Source: CAD feature listing. Evaluate the final solid. Frame: model axes, mm. A direction names the side the tool comes from. Give positions to 0.01 mm unless a question says otherwise; leave off trailing zeros. Order: outer loops, then holes, each group sorted by start corner. A loop starts at its lowest first (then second) coordinate and runs counter-clockwise, first axis right, second up. Notation, with made-up numbers: M 20,48 L 53,48 A27 ccw 53,76 Z; hole C 69.5,-14.75 d9. An arc over 180 degrees is marked long. Return JSON: item names as keys, results as strings.
from build123d import *

# Parameters (mm, degrees)
F1_DEPTH     = 25.4
F2_T         = -2.54
F3_T4_DEPTH  = 109.6353324848
F3_T9_DEPTH  = 109.6353324848
F3_T14_DEPTH = 38.5537016023
F3_T19_DEPTH = 38.5537016023
F3_T24_DEPTH = 109.6353324848
F3_T29_DEPTH = 38.5537016023
F3_T34_DEPTH = 109.6353324848
F3_T39_DEPTH = 38.5537016023
F4_W         = 7.5721852481
F4_H         = 7.5721852481
F5_DEPTH     = 50.8
F6_SIZE      = 5.08
F7_R         = 5.08


# Not quite as in the source:
# - a fillet or chamfer that OpenCascade refuses, or shapes differently, is made with other operations: its cross-section is extruded or revolved along the edge and cut away or added


with BuildPart() as f1:
    # F0 (on Front) → F1 (new body)
    with BuildSketch(Plane.XZ):
        Polygon((-50.8, -50.8), (50.8, -50.8), (50.8, 50.8), (32.1275666356, 46.4897789061), (20.0797300786, -40.3164364398), (-20.0797300786, -40.3164364398), (-32.1275666356, 46.4897789061), (-50.8, 50.8), align=None)
    extrude(amount=F1_DEPTH)

    # F2
    f2_openings = [f1.faces().sort_by_distance(p)[0] for p in [
        (-41.463783, -12.7, 48.644889),
        (-26.103648, -12.7, 3.086671),
        (0, -12.7, -40.316436),
        (41.463783, -12.7, 48.644889),
        (26.103648, -12.7, 3.086671),
    ]]
    offset(amount=F2_T, openings=f2_openings)

    # F3: fillet of radius 5.08 on 8 edges, made by hand


with BuildPart() as f3_tool2:
    # F3_s3 → F3_t4 (new body)
    with BuildSketch(Plane(origin=(8.4495366949, 0, 60.8800010222), x_dir=(0, 1, 0), z_dir=(-0.1374722959, 0, -0.9905056122))):
        with BuildLine():
            ThreePointArc((0, 25.4314784161), (-1.8594090512, 27.2908874673), (-2.54, 29.8308874673))
            Line((-2.54, 29.8308874673), (-2.54, 25.4314784161))
            Line((-2.54, 25.4314784161), (0, 25.4314784161))
        make_face()
    extrude(amount=F3_T4_DEPTH)

    split(bisect_by=Plane.XY.offset(-40.3164364398), keep=Keep.TOP)


with BuildPart() as f1_1:
    add(f1.part)

    # F3_t1: cut F3_tool2
    add(f3_tool2.part, mode=Mode.SUBTRACT)


with BuildPart() as f3_tool7:
    # F3_s8 → F3_t9 (new body)
    with BuildSketch(Plane(origin=(6.6222841773, 0, -47.7144111022), x_dir=(0, 1, 0), z_dir=(-0.1374722959, 0, 0.9905056122))):
        with BuildLine():
            ThreePointArc((0, 25.4314784161), (-1.8594090512, 27.2908874673), (-2.54, 29.8308874673))
            Line((-2.54, 29.8308874673), (-2.54, 25.4314784161))
            Line((-2.54, 25.4314784161), (0, 25.4314784161))
        make_face()
    extrude(amount=F3_T9_DEPTH)

    split(bisect_by=Plane.XY.offset(-40.3164364398), keep=Keep.TOP)


with BuildPart() as f1_2:
    add(f1_1.part)

    # F3_t6: cut F3_tool7
    add(f3_tool7.part, mode=Mode.SUBTRACT)


with BuildPart() as f3_tool12:
    # F3_s13 → F3_t14 (new body)
    with BuildSketch(Plane(origin=(67.5399359806, 0, 15.5904723858), x_dir=(0, 1, 0), z_dir=(-0.9743774967, 0, -0.2249188607))):
        with BuildLine():
            ThreePointArc((0, -38.0724987065), (-1.8594090512, -36.2130896553), (-2.54, -33.6730896553))
            Line((-2.54, -33.6730896553), (-2.54, -38.0724987065))
            Line((-2.54, -38.0724987065), (0, -38.0724987065))
        make_face()
    extrude(amount=F3_T14_DEPTH)

    split(bisect_by=Plane.YZ.offset(48.26), keep=Keep.BOTTOM)


with BuildPart() as f1_3:
    add(f1_2.part)

    # F3_t11: cut F3_tool12
    add(f3_tool12.part, mode=Mode.SUBTRACT)


with BuildPart() as f3_tool17:
    # F3_s18 → F3_t19 (new body)
    with BuildSketch(Plane(origin=(-29.9740767247, 0, 6.9190177438), x_dir=(0, 1, 0), z_dir=(-0.9743774967, 0, 0.2249188607))):
        with BuildLine():
            ThreePointArc((0, -38.0724987065), (-1.8594090512, -36.2130896553), (-2.54, -33.6730896553))
            Line((-2.54, -33.6730896553), (-2.54, -38.0724987065))
            Line((-2.54, -38.0724987065), (0, -38.0724987065))
        make_face()
    extrude(amount=F3_T19_DEPTH)

    split(bisect_by=Plane.YZ.offset(-48.26), keep=Keep.TOP)


with BuildPart() as f1_4:
    add(f1_3.part)

    # F3_t16: cut F3_tool17
    add(f3_tool17.part, mode=Mode.SUBTRACT)


with BuildPart() as f3_tool22:
    # F3_s23 → F3_t24 (new body)
    with BuildSketch(Plane(origin=(6.6222841773, 0, -47.7144111022), x_dir=(0, 1, 0), z_dir=(-0.1374722959, 0, 0.9905056122))):
        with BuildLine():
            ThreePointArc((-25.4, 25.4314784161), (-23.5405909488, 27.2908874673), (-22.86, 29.8308874673))
            Line((-22.86, 29.8308874673), (-22.86, 25.4314784161))
            Line((-22.86, 25.4314784161), (-25.4, 25.4314784161))
        make_face()
    extrude(amount=F3_T24_DEPTH)

    split(bisect_by=Plane.XY.offset(-40.3164364398), keep=Keep.TOP)


with BuildPart() as f1_5:
    add(f1_4.part)

    # F3_t21: cut F3_tool22
    add(f3_tool22.part, mode=Mode.SUBTRACT)


with BuildPart() as f3_tool27:
    # F3_s28 → F3_t29 (new body)
    with BuildSketch(Plane(origin=(-29.9740767247, 0, 6.9190177438), x_dir=(0, 1, 0), z_dir=(-0.9743774967, 0, 0.2249188607))):
        with BuildLine():
            ThreePointArc((-25.4, -38.0724987065), (-23.5405909488, -36.2130896553), (-22.86, -33.6730896553))
            Line((-22.86, -33.6730896553), (-22.86, -38.0724987065))
            Line((-22.86, -38.0724987065), (-25.4, -38.0724987065))
        make_face()
    extrude(amount=F3_T29_DEPTH)

    split(bisect_by=Plane.YZ.offset(-48.26), keep=Keep.TOP)


with BuildPart() as f1_6:
    add(f1_5.part)

    # F3_t26: cut F3_tool27
    add(f3_tool27.part, mode=Mode.SUBTRACT)


with BuildPart() as f3_tool32:
    # F3_s33 → F3_t34 (new body)
    with BuildSketch(Plane(origin=(8.4495366949, 0, 60.8800010222), x_dir=(0, 1, 0), z_dir=(-0.1374722959, 0, -0.9905056122))):
        with BuildLine():
            ThreePointArc((-25.4, 25.4314784161), (-23.5405909488, 27.2908874673), (-22.86, 29.8308874673))
            Line((-22.86, 29.8308874673), (-22.86, 25.4314784161))
            Line((-22.86, 25.4314784161), (-25.4, 25.4314784161))
        make_face()
    extrude(amount=F3_T34_DEPTH)

    split(bisect_by=Plane.XY.offset(-40.3164364398), keep=Keep.TOP)


with BuildPart() as f1_7:
    add(f1_6.part)

    # F3_t31: cut F3_tool32
    add(f3_tool32.part, mode=Mode.SUBTRACT)


with BuildPart() as f3_tool37:
    # F3_s38 → F3_t39 (new body)
    with BuildSketch(Plane(origin=(67.5399359806, 0, 15.5904723858), x_dir=(0, 1, 0), z_dir=(-0.9743774967, 0, -0.2249188607))):
        with BuildLine():
            ThreePointArc((-25.4, -38.0724987065), (-23.5405909488, -36.2130896553), (-22.86, -33.6730896553))
            Line((-22.86, -33.6730896553), (-22.86, -38.0724987065))
            Line((-22.86, -38.0724987065), (-25.4, -38.0724987065))
        make_face()
    extrude(amount=F3_T39_DEPTH)

    split(bisect_by=Plane.YZ.offset(48.26), keep=Keep.BOTTOM)


with BuildPart() as f1_8:
    add(f1_7.part)

    # F3_t36: cut F3_tool37
    add(f3_tool37.part, mode=Mode.SUBTRACT)

    # F4 (on Front) → F5 (join)
    with BuildSketch(Plane.XZ):
        Polygon((-73.3337104321, -50.8196800947), (-54.8367798328, -50.8196800947), (-54.8367798328, -43.2474948466), (-47.2645945847, -43.2474948466), (-47.2645945847, -30.0912298262), (-73.3337104321, -30.0912298262), align=None)
        with Locations((-51.0506872088, -47.0335874707)):
            Rectangle(F4_W, F4_H)
    extrude(amount=F5_DEPTH)

    # F6
    f6_edges = [f1_8.edges().sort_by_distance(p)[0] for p in [
        (-50.8, -12.7, -30.09123),
    ]]
    chamfer(f6_edges, length=F6_SIZE)

    # F7
    f7_edges = [f1_8.edges().sort_by_distance(p)[0] for p in [
        (-73.33371, -25.4, -30.09123),
        (-60.299153, -50.8, -50.81968),
    ]]
    fillet(f7_edges, radius=F7_R)


solid = f1_8.part
1. First-contact query: pin 1 (5 mm diameter, centred on x = 36, y = -29, fed in from -Z); pin 2 (7.5 mm diameter, centred on x = -17.5, y = -16, fed in from -Z); pin 3 (2 mm diameter, centred on x = -0.5, y = -2, fed in from +Z); pin 4 (2 mm diameter, centred on x = -25, y = -15, fed in from +Z). Flat tips, straight axial feed; report the tip coordinate or a pass-through.
Evaluation:
{"pin 1": "passes through", "pin 2": "stops at z = -50.8", "pin 3": "stops at z = -40.32", "pin 4": "stops at z = -48.26"}
2. Set-up query: faces 1 (the face through (0, -13, -48.26)), 2 (the face through (-26, 0, -11)), 3 (the face through (49.5, -12.5, 50.5)). Return all of +Z, -Z, +X, -X, +Y, -Y with unobstructed straight access to the full face (end or side cutting, diameter ignored); none if empty.
Evaluation:
{"face 1": "+Z", "face 2": "+Z, -Z, +X, -X, +Y", "face 3": "+Z, +Y, -Y"}
3. Ray query, probe 1 along Y at (x, z) = (-48, 40); probe 2 along X at (y, z) = (-17.5, -23.5); probe 3 along Z at (x, y) = (-67.5, -41). Return the intervals inside material, ascending.
Evaluation:
{"probe 1": "y = -25.4 to -22.86, -2.54 to 0", "probe 2": "x = -50.8 to -48.26, 48.26 to 50.8", "probe 3": "z = -50.82 to -30.09"}
4. Section query C-C (y = -27.5). Return loops of the section in (x, z).
Evaluation:
{"outline": "M -73.33,-50.82 L -47.26,-50.82 L -47.26,-30.09 L -68.25,-30.09 A5.08 ccw -73.33,-35.17 Z"}
5. Section query B-B (x = 3). Return loops of the section in (y, z).
Evaluation:
{"outline": "M -25.4,-50.8 L 0,-50.8 L 0,-40.32 L -2.54,-40.32 L -2.54,-48.26 L -22.86,-48.26 L -22.86,-40.32 L -25.4,-40.32 Z"}
6. Draft query along X for faces 4 (the face through (0, -1, -40.316)), 5 (the face through (-60, -31, -30.091)), 6 (the face through (-50.8, -13, 13)). Return one class per face: pulls with the +X half, pulls with the -X half, needs draft (parallel to the pull), parting line crosses it, or undercut.
Evaluation:
{"face 4": "undercut", "face 5": "needs draft", "face 6": "pulls with the -X half"}
